```python
from build123d import *

# Parameters (mm, degrees)
SKETCH1_W             = 28
SKETCH1_H             = 28
BOSS_EXTRUDE1_DEPTH   = 1
SKETCH2_R             = 9
BOSS_EXTRUDE2_DEPTH   = 0.5
F_4_CLEARANCE_HOLE1_D = 2.9464


with BuildPart() as part:
    # Sketch1 → Boss-Extrude1 (new body)
    with BuildSketch(Plane.XY):
        Rectangle(SKETCH1_W, SKETCH1_H)
    extrude(amount=BOSS_EXTRUDE1_DEPTH)

    # Sketch2 → Boss-Extrude2 (add)
    with BuildSketch(Plane.XY.offset(1)):
        Circle(SKETCH2_R)
    extrude(amount=BOSS_EXTRUDE2_DEPTH)

    # #4 Clearance Hole1 (through all)
    with Locations(Plane.XY.offset(1)):
        with Locations((11.4, -11.4), (-11.4, 11.4)):
            Hole(F_4_CLEARANCE_HOLE1_D / 2)


solid = part.part
```
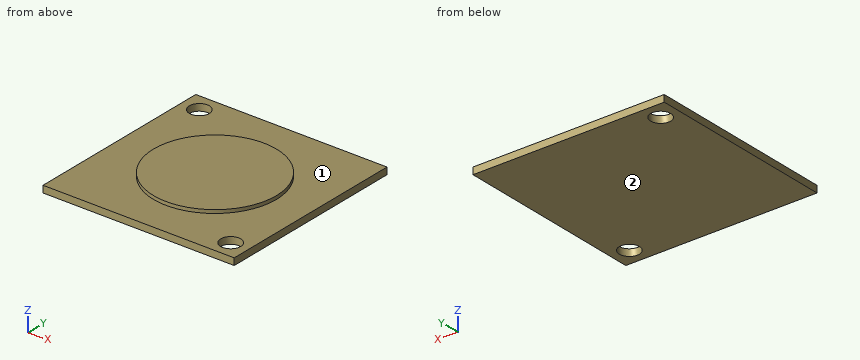
Geometry check sheet. Reference: the model listing, model coordinates, mm. Face numbers are marked on the shaded views. A direction names the side the tool comes from. Give positions to 0.01 mm unless a question says otherwise; leave off trailing zeros. Loops run counter-clockwise (first coordinate to the right, second up) from the corner with the lowest first, then second, coordinate; pieces in that order, holes last. Notation, with made-up numbers: M 58,49 L 107,49 A29 cw 107,77 Z; hole C 38,55.25 d2. An arc over 180 degrees is marked long. Write item = value, one per line. Start each with the question number.
1. Thickness scan on probe 1 along Y at (x, z) = (11.4, 0.6); probe 2 along Y at (x, z) = (10.5, 0.7); probe 3 along Z at (x, y) = (9.25, 0.5). Record the ranges inside material, lowest first.
2. Section check B-B, the plane x = 11.4. Enter the section's corners in (y, z), plus the area to 3 significant figures.
3. Go/stop test with flat-tipped pins: P1, Ø3.5, axis at x = 11.4, y = -11.4, coming from the +Z side; P2, Ø1.8, axis at x = -11.4, y = 11.4, coming from the +Z side. Record where each tip stops, or that it passes through.
4. Tool access check on the marked faces 1 and 2. Record the directions out of +Z, -Z, +X, -X, +Y, -Y that give a thin tool (end or side, any length) a straight path to the whole face; none if there is none.
5. Section check A-A, the plane y = -11.4. Enter the section's corners in (x, z).
6. Section check C-C, the plane z = 0.7. Enter the section's corners in (x, y), plus the area to 3 significant figures.
7. Section check D-D, the plane y = 0. Enter the section's corners in (x, z), plus the area to 3 significant figures.
Values follow:
q1.probe_1 = -14 to -12.87, -9.93 to 14
q1.probe_2 = -14 to -12.57, -10.23 to 14
q1.probe_3 = 0 to 1
q2.outline = M -14,0 L -12.87,0 L -12.87,1 L -14,1 Z; M -9.93,0 L 14,0 L 14,1 L -9.93,1 Z
q2.area = 25.1 mm^2
q3.P1 = 1
q3.P2 = through
q4.face_1 = +Z
q4.face_2 = -Z, +X, -X, +Y, -Y
q5.outline = M -14,0 L 9.93,0 L 9.93,1 L -14,1 Z; M 12.87,0 L 14,0 L 14,1 L 12.87,1 Z
q6.outline = M -14,-14 L 14,-14 L 14,14 L -14,14 Z; hole C -11.4,11.4 d2.95; hole C 11.4,-11.4 d2.95
q6.area = 770 mm^2
q7.outline = M -14,0 L 14,0 L 14,1 L 9,1 L 9,1.5 L -9,1.5 L -9,1 L -14,1 Z
q7.area = 37.0 mm^2
